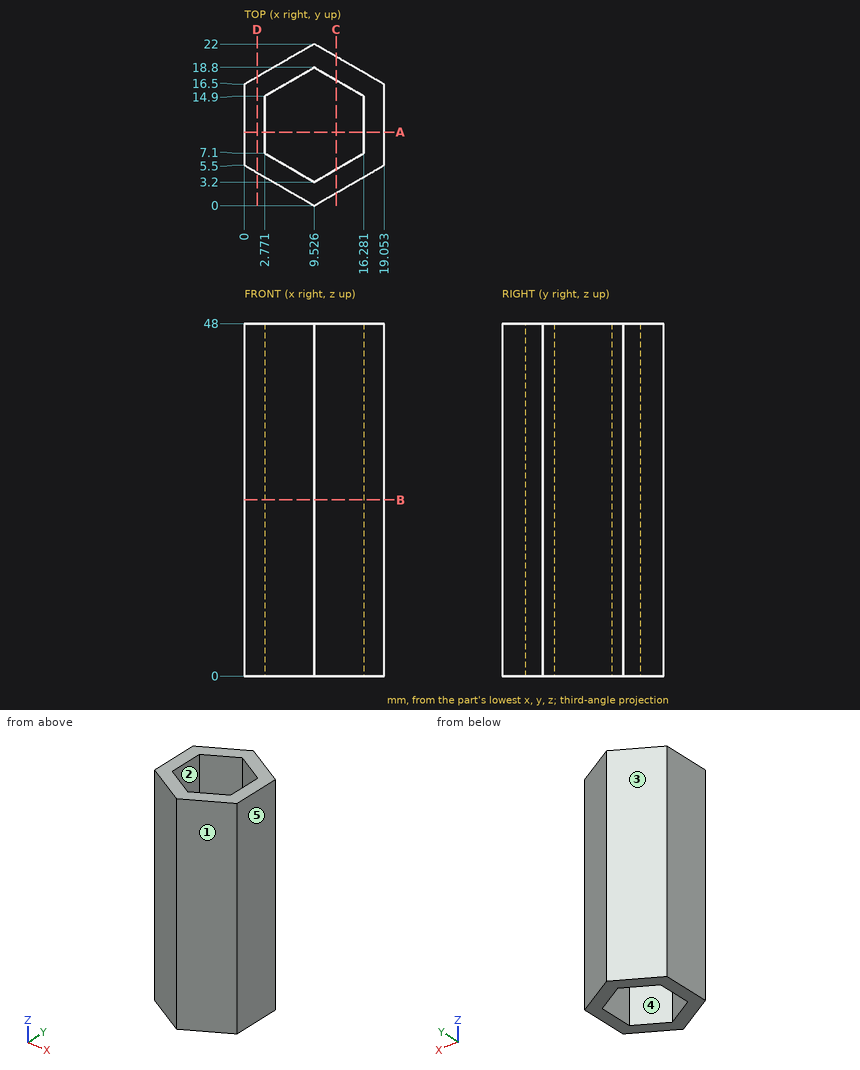
Print and shaded views of the part. All mm, measured from the part's lowest x, y and z. A direction names the side the tool comes from. Give positions to 0.01 mm unless a question says otherwise; leave off trailing zeros. Loops run counter-clockwise (first coordinate to the right, second up) from the corner with the lowest first, then second, coordinate; pieces in that order, holes last. Notation, with made-up numbers: M 49,25 L 100,25 A26 ccw 100,46 Z; hole C 89.25,51 d10. An arc over 180 degrees is marked long. Write each question's results on one line, items separated by ' | '.
Q1. Band-saw the part on A-A on y = 10. Write the cut outline in (x, z), and give its area (3 significant figures).
Geometry check:
outline: M 0,0 L 2.77,0 L 2.77,48 L 0,48 Z; M 16.28,0 L 19.05,0 L 19.05,48 L 16.28,48 Z | area: 266 mm²
Q2. Which spindle directions (+Z, -Z, +X, -X, +Y, -Y) get a long thin tool onto all of the face, cutting with end or side? Do the marked faces 4 and 5. Say none if no direction does.
Geometry check:
face 4: +Z, -Z | face 5: +Z, -Z, +X, +Y, -Y
Q3. Flat gauge pins, fed straight in: P1, Ø1.5, axis at x = 7.5, z = 14, coming from the -Y side; P2, Ø6, axis at x = 17, z = 34.5, coming from the +Y side; P3, Ø4, axis at x = 7, z = 40.5, coming from the +Y side (1 decimal). Where does each tip first touch, or does it go through?
Geometry check:
P1: stops at y = 0.74 | P2: stops at y = 19.42 | P3: stops at y = 21.7
Q4. Mould opens along Y. For the marked faces 1, 2 and 3 say: pulls with the +Y half, pulls with the -Y half, needs draft (parallel to the pull), parting line crosses it, or undercut.
Geometry check:
face 1: pulls with the -Y half | face 2: undercut | face 3: pulls with the +Y half
Q5. Probe probe 1 along X at (y, z) = (10.75, 31); probe 2 along Y at (x, z) = (4.25, 35.5) (1 decimal); probe 3 along Y at (x, z) = (8.75, 6). List the from-to ranges inside material, lowest first.
Geometry check:
probe 1: x = 0 to 2.77, 16.28 to 19.05 | probe 2: y = 3 to 6.2, 15.8 to 19 | probe 3: y = 0.45 to 3.65, 18.35 to 21.55
Q6. Band-saw the part on B-B on z = 24. Write the cut outline in (x, y).
Geometry check:
outline: M 0,5.5 L 9.53,0 L 19.05,5.5 L 19.05,16.5 L 9.53,22 L 0,16.5 Z; hole M 2.77,7.1 L 9.53,3.2 L 16.28,7.1 L 16.28,14.9 L 9.53,18.8 L 2.77,14.9 Z
Q7. Band-saw the part on D-D on x = 1.75. Write the cut outline in (y, z).
Geometry check:
outline: M 4.49,0 L 17.51,0 L 17.51,48 L 4.49,48 Z
Q8. Band-saw the part on C-C on x = 12.5. Write the cut outline in (y, z).
Geometry check:
outline: M 1.72,0 L 4.92,0 L 4.92,48 L 1.72,48 Z; M 17.08,0 L 20.28,0 L 20.28,48 L 17.08,48 Z
